Check sheet for the modelled part. Datum: model origin and axes. Units: mm. A direction names the side the tool comes from. Round coordinates to 2 decimals unless told otherwise and drop trailing zeros. Write each loop counter-clockwise with the first axis right and the second up, starting at its lowest first coordinate (ties: lowest second). Pieces come first, ordered by that corner, then holes. Notation, with made-up numbers: (85, -9) -> (140, -9) arc R13 ccw to (140, 14) -> close; hole circle Ø3 at (24, 7.25). An arc over 180 degrees is marked (long way). One line per item, written item: value.
from build123d import *

# Parameters (mm, degrees)
ESBO_O1_W                = 94
ESBO_O1_H                = 37
RESSALTO_EXTRUS_O1_DEPTH = 3
ESBO_O2_W                = 82
ESBO_O2_H                = 3.2
ESBO_O2_W_2              = 3.2
ESBO_O2_H_2              = 18
CORTE_EXTRUS_O2_DEPTH    = 3
ESBO_O2_5_R              = 1.1
ESBO_O2_5_W              = 82
ESBO_O2_5_H              = 3.2
ESBO_O2_5_W_2            = 3.2
ESBO_O2_5_H_2            = 18
ESBO_O2_5_W_3            = 23
ESBO_O2_5_H_3            = 12
CORTE_EXTRUS_O4_DEPTH    = 10


with BuildPart() as part:
    # Esbo_o1 → Ressalto-extrus_o1 (new body)
    with BuildSketch(Plane(origin=(0, 0, 0), x_dir=(1, 0, 0), z_dir=(0, 1, 0))):
        with Locations((15.423867314, 16.168005002)):
            Rectangle(ESBO_O1_W, ESBO_O1_H)
    extrude(amount=RESSALTO_EXTRUS_O1_DEPTH)

    # Esbo_o2 → Corte-extrus_o2 (cut)
    with BuildSketch(Plane(origin=(0, 3, 0), x_dir=(1, 0, 0), z_dir=(0, 1, 0))):
        with Locations((15.423867314, 3.918005002)):
            Rectangle(ESBO_O2_W, ESBO_O2_H)
        with Locations((15.423867314, 28.418005002)):
            Rectangle(ESBO_O2_W, ESBO_O2_H)
        with Locations((-27.176132686, 16.168005002)):
            Rectangle(ESBO_O2_W_2, ESBO_O2_H_2)
    extrude(amount=-CORTE_EXTRUS_O2_DEPTH, mode=Mode.SUBTRACT)

    # Esbo_o2_5 → Corte-extrus_o4 (cut)
    with BuildSketch(Plane(origin=(0, 3, 0), x_dir=(1, 0, 0), z_dir=(0, 1, 0))):
        with Locations(Location((5.983867314, 16.168005002, 0), (0, 0, 270))):
            Circle(ESBO_O2_5_R)
        with Locations(Location((-22.136132686, 16.168005002, 0), (0, 0, 270))):
            Circle(ESBO_O2_5_R)
        with Locations(Location((52.25559416, 15.786516757, 0), (0, 0, 270))):
            Circle(ESBO_O2_5_R)
        with Locations(Location((24.13559416, 15.786516757, 0), (0, 0, 270))):
            Circle(ESBO_O2_5_R)
        with Locations((15.423867314, 3.918005002)):
            Rectangle(ESBO_O2_5_W, ESBO_O2_5_H)
        with Locations((15.423867314, 28.418005002)):
            Rectangle(ESBO_O2_5_W, ESBO_O2_5_H)
        with Locations((-27.176132686, 16.168005002)):
            Rectangle(ESBO_O2_5_W_2, ESBO_O2_5_H_2)
        with Locations((-8.076132686, 16.168005002)):
            Rectangle(ESBO_O2_5_W_3, ESBO_O2_5_H_3)
        with Locations((58.023867314, 16.168005002)):
            Rectangle(ESBO_O2_5_W_2, ESBO_O2_5_H_2)
        with Locations((38.19559416, 16.196023894)):
            Rectangle(ESBO_O2_5_W_3, ESBO_O2_5_H_3)
    extrude(amount=-CORTE_EXTRUS_O4_DEPTH, mode=Mode.SUBTRACT)


solid = part.part
Item 1: Material ranges on line 1 along Z through (x, y) = (-22, 1.55); line 2 along Z through (x, y) = (-14, 1.45); line 3 along Z through (x, y) = (13.5, 1.7), recorded low to high.
Result set:
line 1: -34.67 to -30.02, -26.82 to -17.26, -15.08 to -5.52, -2.32 to 2.33
line 2: -34.67 to -30.02, -26.82 to -22.17, -10.17 to -5.52, -2.32 to 2.33
line 3: -34.67 to -30.02, -26.82 to -5.52, -2.32 to 2.33
Item 2: Sectioned sample at B-B (x = 13). Enter the section's corners in (y, z).
Result set:
outline: (0, -34.67) -> (3, -34.67) -> (3, -30.02) -> (0, -30.02) -> close; (0, -26.82) -> (3, -26.82) -> (3, -5.52) -> (0, -5.52) -> close; (0, -2.32) -> (3, -2.32) -> (3, 2.33) -> (0, 2.33) -> close
Item 3: Sectioned sample at C-C (y = 2.2). State how many separate pieces and enclosed holes the cut face has, then the cut area to 3 significant figures.
Result set:
separate pieces: 1
enclosed holes: 10
area: 2,270 mm^2
Item 4: Release check for a two-part mould opening along X. For faces 3 (the flat face through (15, 2, -2.318)), 4 (the flat face through (15, 1, 2.332)), 5 (the flat face through (62.424, 1, -16)), 6 (the flat face through (-27, 2, -25.168)) record: pulls with the +X half, pulls with the -X half, needs draft (parallel to the pull), parting line crosses it, or undercut.
Result set:
face 3: undercut
face 4: needs draft
face 5: pulls with the +X half
face 6: undercut
Item 5: Tool access check on faces 1 (the flat face through (15, 3, -16)), 2 (the flat face through (-8, 2, -22.168)). Record the directions out of +Z, -Z, +X, -X, +Y, -Y that give a thin tool (end or side, any length) a straight path to the whole face; none if there is none.
Result set:
face 1: +Z, -Z, +X, -X, +Y
face 2: +Y, -Y
Item 6: Sectioned sample at A-A (x = 40.5). Enter the section's corners in (y, z).
Result set:
outline: (0, -34.67) -> (3, -34.67) -> (3, -30.02) -> (0, -30.02) -> close; (0, -26.82) -> (3, -26.82) -> (3, -22.2) -> (0, -22.2) -> close; (0, -10.2) -> (3, -10.2) -> (3, -5.52) -> (0, -5.52) -> close; (0, -2.32) -> (3, -2.32) -> (3, 2.33) -> (0, 2.33) -> close
